Check sheet for the modelled part. Datum: model origin and axes. Units: mm. A direction names the side the tool comes from. Round coordinates to 2 decimals unless told otherwise and drop trailing zeros. Write each loop counter-clockwise with the first axis right and the second up, starting at its lowest first coordinate (ties: lowest second). Pieces come first, ordered by that corner, then holes. Notation, with made-up numbers: M -33.5,-4.75 L -22.5,-4.75 A20 cw -22.5,8.25 Z; hole C -38,-32 d9. An arc over 180 degrees is marked long. One line per item, written item: value.
Autodesk Inventor part; units mm, degrees
ref_plane "Plano de trabajo1" through (75, 0, 0) normal (1, 0, 0) x (0, 0, -1)
ref_plane "Plano de trabajo2" through (150, 25, 68) normal (0, 0, 1) x (1, 0, 0)
ref_plane "Plano de trabajo3" through (75, 0, 0) normal (1, 0, 0) x (0, 0, -1)
sketch "Boceto1" plane through (0, 0, 0) normal (0, 0, 1) x (1, 0, 0)
  line L0 (0, 0) -> (150, 0)
  line L1 (150, 0) -> (150, 150)
  line L2 (150, 150) -> (0, 150)
  line L3 (0, 150) -> (0, 0)
  line L4 (5, 145) -> (145, 145)
  line L5 (145, 145) -> (145, 5)
  line L6 (145, 5) -> (5, 5)
  line L7 (5, 5) -> (5, 145)
  dimension "d0" = 150
  dimension "d1" = 150
  dimension "d2" = 5
extrude "Extrusión1" add sketch "Boceto1" along normal blind 150
sketch "Boceto2" plane through (150, 0, 0) normal (1, 0, 0) x (0, 0, -1)
  line L0 (-150, 0) -> (-150, 150)
  line L1 (-150, 75) -> (-190, 75) construction
  line L2 (-190, 75) -> (-150, 150)
  line L3 (0, 0) -> (-150, 0) construction
  line L4 (-150, 0) -> (-190, 75)
  dimension "d5" = 40
extrude "Extrusión2" add sketch "Boceto2" against normal blind 5
ref_plane "Plano de trabajo1" through (75, 0, 0) normal (1, 0, 0) x (0, 0, -1)
mirror "Simetría1" about plane through (75, 0, 0) normal (1, 0, 0) of "Extrusión2"
sketch "Boceto3" plane through (0, 150, 0) normal (0, 1, 0) x (1, 0, 0)
  line L0 (105, -60) -> (45, -60)
  line L1 (45, -60) -> (45, -95)
  line L2 (60, -110) -> (90, -110)
  line L3 (105, -95) -> (105, -60)
  line L4 (150, 0) -> (0, 0)
  line L5 (145, -150) -> (5, -150)
  arc A0 (90, -110) -> (105, -95) centre (90, -95) ccw
  arc A1 (45, -95) -> (60, -110) centre (60, -95) ccw
  point P0 (45, -110)
  point P1 (105, -110)
  point P2 (75, -60)
  point P3 (75, 0)
  dimension "d8" = 60
  dimension "d9" = 50
  dimension "d10" = 40
  dimension "d11" = 15
extrude "Extrusión3" cut sketch "Boceto3" against normal through all
sketch "Boceto4" plane through (150, 0, 0) normal (1, 0, 0) x (0, 0, -1)
  line L0 (-13, 20) -> (-123, 20)
  line L1 (-128, 25) -> (-128, 75)
  line L2 (-123, 80) -> (-13, 80)
  line L3 (-8, 75) -> (-8, 25)
  line L4 (0, 0) -> (0, 150)
  line L5 (0, 0) -> (-150, 0)
  arc A0 (-123, 80) -> (-128, 75) centre (-123, 75) ccw
  arc A1 (-8, 75) -> (-13, 80) centre (-13, 75) ccw
  arc A2 (-13, 20) -> (-8, 25) centre (-13, 25) ccw
  arc A3 (-128, 25) -> (-123, 20) centre (-123, 25) ccw
  point P0 (-128, 80)
  point P1 (-128, 20)
  point P2 (-8, 80)
  dimension "d14" = 120
  dimension "d15" = 60
  dimension "d16" = 8
  dimension "d17" = 20
  dimension "d18" = 5
extrude "Extrusión4" cut sketch "Boceto4" against normal up to surface (5 mm away)
sketch "Boceto5" plane through (0, 0, 0) normal (-1, 0, 0) x (0, 0, 1)
  line L0 (65, 125) -> (115, 125)
  line L1 (120, 120) -> (120, 30)
  line L2 (115, 25) -> (65, 25)
  line L3 (60, 30) -> (60, 120)
  line L4 (0, 150) -> (0, 0)
  arc A0 (120, 120) -> (115, 125) centre (115, 120) ccw
  arc A1 (115, 25) -> (120, 30) centre (115, 30) ccw
  arc A2 (65, 125) -> (60, 120) centre (65, 120) ccw
  arc A3 (60, 30) -> (65, 25) centre (65, 30) ccw
  point P0 (60, 150)
  point P1 (120, 25)
  point P2 (120, 125)
  point P3 (60, 25)
  point P4 (60, 75)
  point P5 (0, 75)
  dimension "d21" = 60
  dimension "d22" = 100
  dimension "d23" = 60
  dimension "d24" = 5
extrude "Extrusión5" cut sketch "Boceto5" against normal blind 10
sketch "Boceto6" plane through (150, 0, 0) normal (1, 0, 0) x (0, 0, -1)
  line L0 (-190, 75) -> (-150, 0)
  line L1 (-150, 150) -> (-190, 75)
  line L2 (-154.4118, 152.3529) -> (-195.6667, 75)
  line L3 (-195.6667, 75) -> (-154.4118, -2.3529)
  line L4 (-154.4118, 152.3529) -> (-144.4118, 152.3529)
  line L5 (-144.4118, 152.3529) -> (-144.4118, 150)
  line L6 (-154.4118, -2.3529) -> (-144.4118, -2.3529)
  line L7 (-144.4118, -2.3529) -> (-144.4118, 0)
  line L8 (0, 0) -> (-150, 0)
  line L9 (0, 150) -> (-150, 150)
  dimension "d27" = 5
  dimension "d28" = 10
extrude "Extrusión6" add sketch "Boceto6" along normal blind 10 and the other way blind 160
fillet "Empalme1" radius 5 3 edges at (75, 152.3529, 154.4118) (75, 75, 195.6667) (75, -2.3529, 154.4118)
sketch "Boceto7" plane through (150, 25, 8) normal (0, 0, 1) x (1, 0, 0)
  circle A0 centre (-2.5, 2.5) radius 1.25
  line L0 (0, 50) -> (0, 0)
  line L1 (0, 0) -> (-5, 0)
  point P0 (-150, -25)
  point P1 (-2.5, 0)
  dimension "d34" = 2.5
  dimension "d35" = 2.5
  dimension "d36" = 2.5
extrude "Extrusión7" cut sketch "Boceto7" against normal blind 3
ref_plane "Plano de trabajo2" through (150, 25, 68) normal (0, 0, 1) x (1, 0, 0)
mirror "Simetría2" about plane through (150, 25, 68) normal (0, 0, 1) of "Extrusión7"
sketch "Boceto8" plane through (160, 0, 0) normal (1, 0, 0) x (0, 0, -1)
  arc A0 (-155.8235, 0.2941) -> (-151.4118, -2.3529) centre (-151.4118, 2.6471) ccw
  line L0 (-151.4118, -2.3529) -> (-144.4118, -2.3529)
  line L1 (-144.4118, -2.3529) -> (-144.4118, 0)
  line L2 (-144.4118, 0) -> (-150, 0)
  line L3 (-150, 0) -> (-190, 75)
  line L4 (-190, 75) -> (-150, 150)
  line L5 (-150, 150) -> (-144.4118, 150)
  line L6 (-144.4118, 150) -> (-144.4118, 152.3529)
  line L7 (-144.4118, 152.3529) -> (-151.4118, 152.3529)
  arc A1 (-151.4118, 152.3529) -> (-155.8235, 149.7059) centre (-151.4118, 147.3529) ccw
  line L8 (-155.8235, 149.7059) -> (-194.4118, 77.3529)
  arc A2 (-194.4118, 77.3529) -> (-194.4118, 72.6471) centre (-190, 75) ccw
  line L9 (-194.4118, 72.6471) -> (-155.8235, 0.2941)
  point P0 (0, 0)
extrude "Extrusión8" cut sketch "Boceto8" against normal through all
sketch "Boceto9" plane through (145, 0, 150) normal (0, -0.4705882, 0.8823529) x (1, 0, 0)
  circle A0 centre (2.5, 2.5) radius 1.5
  line L0 (5, 85) -> (5, 0)
  line L1 (5, 0) -> (0, 0)
  point P0 (-145, -70.5882)
  dimension "d41" = 3
  dimension "d42" = 2.5
  dimension "d43" = 2.5
ref_plane "Plano de trabajo3" through (75, 0, 0) normal (1, 0, 0) x (0, 0, -1)
ref_plane "Plano de trabajo4" through (0, 75, 0) normal (0, -1, 0) x (1, 0, 0)
mirror "Simetría4" about plane through (0, 75, 0) normal (0, -1, 0) of "Extrusión8"
sketch "Boceto10" plane through (0, 150, 0) normal (0, 1, 0) x (1, 0, 0)
  line L0 (5, -115) -> (5, -65)
  arc A0 (45, -95) -> (60, -110) centre (60, -95) ccw
  line L1 (45, -95) -> (45, -60)
  line L2 (45, -60) -> (105, -60)
  line L3 (105, -60) -> (105, -95)
  arc A1 (90, -110) -> (105, -95) centre (90, -95) ccw
  line L4 (90, -110) -> (60, -110)
  line L5 (150, 0) -> (150, -150)
  line L6 (150, 0) -> (0, 0)
  line L7 (0, 0) -> (0, -150)
  line L8 (5, -150) -> (0, -150)
  line L9 (145, -150) -> (5, -150)
  line L10 (150, -150) -> (145, -150)
extrude "Extrusión10" cut sketch "Boceto10" against normal up to surface (145 mm away)
sketch "Boceto11" plane through (150, 0, 150) normal (1, 0, 0) x (0, 0, -1)
  line L0 (0, 0) -> (0, 5)
  line L1 (0, 5) -> (0, 150)
  line L2 (-40, 75) -> (0, 0)
  line L3 (0, 150) -> (-40, 75)
  point P0 (150, 0)
extrude "Extrusión11" cut sketch "Boceto11" against normal through all
sketch "Boceto12" plane through (150, 0, 0) normal (1, 0, 0) x (0, 0, -1)
  circle A0 centre (-147.5, 2.5) radius 1.5
  line L0 (0, 5) -> (-150, 5)
  line L1 (-150, 5) -> (-150, 0)
  line L2 (-75, 5) -> (-75, -25.1445) construction
  circle A1 centre (-2.5, 2.5) radius 1.5
  point P0 (0, 0)
  dimension "d50" = 3
  dimension "d51" = 2.5
  dimension "d52" = 2.5
extrude "Extrusión12" cut sketch "Boceto12" against normal blind 5
mirror "Simetría5" about plane through (75, 0, 0) normal (1, 0, 0) of "Extrusión12"
properties part number "CasaJugueteAPM" material "Plástico ABS"
Q1. Access from +Z, -Z, +X, -X, +Y, -Y to the whole of each face (thin tool, end or side, straight path). Record for faces 4 (the flat face through (76, 2, 150)), 5 (the cylindrical face through (100.49, 2.53, 105.72)).
Completed:
face 4: +Z, +X, -X, +Y, -Y
face 5: +Y, -Y
Q2. Sectioned sample at B-B on y = 2.5. Enter the section's corners in (x, z), and give its area (3 significant figures).
Completed:
outline: M 0,0 L 150,0 L 150,1 L 145,1 L 145,4 L 150,4 L 150,146 L 145,146 L 145,149 L 150,149 L 150,150 L 0,150 L 0,149 L 5,149 L 5,146 L 0,146 L 0,4 L 5,4 L 5,1 L 0,1 Z; hole M 45,60 L 105,60 L 105,95 A15 ccw 90,110 L 60,110 A15 ccw 45,95 Z
area: 19,500 mm^2
Q3. Sectioned sample at C-C on z = 98.5. Enter the section's corners in (x, y), and give its area (3 significant figures).
Completed:
outline: M 0,0 L 45.41,0 L 45.41,5 L 0,5 Z; M 104.59,0 L 150,0 L 150,5 L 104.59,5 Z
area: 454 mm^2
Q4. Depth check by flat-ended pin: P1, Ø2.5, axis at y = 2.5, z = 2.5, coming from the +X side; P2, Ø0.9, axis at y = 3, z = 2, coming from the -X side. Enter the tip coordinate at first touch or a pass-through.
Completed:
P1: x = 145
P2: x = 5
Q5. Sectioned sample at A-A on x = 80. Enter the section's corners in (y, z), and give its area (3 significant figures).
Completed:
outline: M 0,0 L 5,0 L 5,60 L 0,60 Z; M 0,110 L 5,110 L 5,150 L 0,150 Z
area: 500 mm^2
Q6. Scan lines: line 1 (X direction, y = 4.05, z = 87.5); line 2 (Y direction, x = 148.8, z = 147.5); line 3 (Z direction, x = 76, y = 2.35). Record each from-to range of solid material in increasing order. Write a range as [from, to].
Completed:
line 1: [0, 45], [105, 150]
line 2: [0, 1], [4, 5]
line 3: [0, 60], [110, 150]
Q7. Draft check along X on faces 1 (the flat face through (0, 3, 74)), 2 (the flat face through (75, 3, 60)), 3 (the flat face through (74, 5, 57)). Enter one of: pulls with the +X half, pulls with the -X half, needs draft (parallel to the pull), parting line crosses it, or undercut.
Completed:
face 1: pulls with the -X half
face 2: undercut
face 3: needs draft
